Work out the finished part from the listing and answer in its coordinate system (mm). A direction names the side the tool comes from. Give positions to 0.01 mm unless a question says otherwise; leave off trailing zeros. Write each loop counter-clockwise with the first axis right and the second up, starting at its lowest first coordinate (ties: lowest second). Pieces come first, ordered by that corner, then holes.
1) A tool of negligible diameter and unlimited length cuts with its end or side. For faces 4 (the face through (-30.426, -17.744, 23.33)), 5 (the face through (-5.357, -7.513, 40.798)), 6 (the face through (0.553, -5.128, -34.887)), from which of +Z, -Z, +X, -X, +Y, -Y can it reach the whole face along a straight path? Write none if from no direction.
2) Given pin 1 Ø1 at (x, y) = (-2, -20.5) entering from -Z; pin 2 Ø3 at (x, y) = (-27, -12.5) entering from +Z; pin 3 Ø24.5 at (x, z) = (-3, -19.5) entering from -Y, each flat-ended and moving along its own axis, determine where each tip first touches the part or whether it passes through.
3) Determine the mould class of faces 1 (the face through (10.19, -16.51, 23.45)), 2 (the face through (-27.24, -20.32, 27.24)), 3 (the face through (-5.357, -22.824, 40.798)) for opening direction Y: pulls with the +Y half, pulls with the -Y half, needs draft (parallel to the pull), parting line crosses it, or undercut.
4) Find section A-A (x = 58). Determine the outline of the cut face in (y, z) (3 decimals), plus the area to 3 significant figures.
5) Straight lines are drawn through the part: probe 1 along Y at (x, z) = (0, -33.5) (3 decimals); probe 2 along Y at (x, z) = (-35.5, 48) (3 decimals); probe 3 along Y at (x, z) = (-23.5, -20.5) (3 decimals). For each, find the intervals that lie inside material, in ascending order.
6) Find section C-C (x = -57.15). Determine the outline of the cut face in (y, z) (3 decimals).
7) Find section B-B (z = 30). Determine the outline of the cut face in (x, y) (3 decimals).
```python
from build123d import *

# Parameters (mm, degrees)
SKETCH1_R                       = 66.675
SKETCH1_R_2                     = 20.32
BOSS_EXTRUDE1_DEPTH             = 4.445
F_1_4_0_25_DIAMETER_HOLE1_D     = 6.35
F_1_4_0_25_DIAMETER_HOLE1_DEPTH = 4.446
CIRPATTERN1_COUNT               = 6
SKETCH6_R                       = 41.148
SKETCH6_R_2                     = 20.32
BOSS_EXTRUDE2_DEPTH             = 25.4
SKETCH9_W                       = 2.9337
SKETCH9_H                       = 5.08
CIRPATTERN2_COUNT               = 6
F_3_32_0_09375_DIAMETER_HOLE1_D = 2.38125
SKETCH13_R                      = 34.925
CUT_EXTRUDE1_DEPTH              = 8.89
CHAMFER2_SIZE                   = 5.08


with BuildPart() as part:
    # Sketch1 → Boss-Extrude1 (new body)
    with BuildSketch(Plane(origin=(0, 0, 0), x_dir=(1, 0, 0), z_dir=(0, 1, 0))):
        Circle(SKETCH1_R)
        Circle(SKETCH1_R_2, mode=Mode.SUBTRACT)
    extrude(amount=BOSS_EXTRUDE1_DEPTH)

    # 1/4 (0.25) Diameter Hole1
    with Locations(Plane(origin=(0, 4.445, 0), x_dir=(1, 0, 0), z_dir=(0, 1, 0))):
        with Locations((57.15, 0)):
            f_1_4_0_25_diameter_hole1 = Hole(F_1_4_0_25_DIAMETER_HOLE1_D / 2, depth=F_1_4_0_25_DIAMETER_HOLE1_DEPTH)

    # CirPattern1: 1/4 (0.25) Diameter Hole1 ×6 about axis
    cirpattern1_axis = Axis((0, 0, 0), (0, 1, 0))
    for i in range(1, CIRPATTERN1_COUNT):
        add(f_1_4_0_25_diameter_hole1.rotate(cirpattern1_axis, i * 360 / CIRPATTERN1_COUNT), mode=Mode.SUBTRACT)

    # Sketch6 → Boss-Extrude2 (add)
    with BuildSketch(Plane.XZ):
        Circle(SKETCH6_R)
        Circle(SKETCH6_R_2, mode=Mode.SUBTRACT)
    extrude(amount=BOSS_EXTRUDE2_DEPTH)

    # Sketch9 → Cut-Revolve3 (revolve, cut)
    with BuildSketch(Plane.XY):
        with Locations((39.80815, -17.78)):
            Rectangle(SKETCH9_W, SKETCH9_H)
    revolve(axis=Axis((0, -0.47625, 0), (0, 1, 0)), mode=Mode.SUBTRACT)

    # Sketch10 → 1/4-20 Tapped Hole1 (revolve, cut)
    with BuildSketch(Plane(origin=(-35.635213315, -7.62, 20.574), x_dir=(0.5, 0, 0.866025404), z_dir=(0, 1, 0))):
        Polygon((0, 0), (0, 14.233816902), (2.5527, 12.7), (2.5527, 0), align=None)
    f_1_4_20_tapped_hole1 = revolve(axis=Axis((-41.134474629, -7.62, 23.749), (0.866025404, 0, -0.5)), mode=Mode.SUBTRACT)

    # CirPattern2: 1/4-20 Tapped Hole1 ×6 about axis
    cirpattern2_axis = Axis((0, -0.47625, 0), (0, 1, 0))
    for i in range(1, CIRPATTERN2_COUNT):
        add(f_1_4_20_tapped_hole1.rotate(cirpattern2_axis, i * 360 / CIRPATTERN2_COUNT), mode=Mode.SUBTRACT)

    # 3/32 (0.09375) Diameter Hole1 (through all)
    with Locations(Plane(origin=(0, 4.445, 0), x_dir=(1, 0, 0), z_dir=(0, 1, 0))):
        with Locations((31.75, 0)):
            Hole(F_3_32_0_09375_DIAMETER_HOLE1_D / 2)

    # Sketch13 → Cut-Extrude1 (cut)
    with BuildSketch(Plane.XZ.offset(25.4)):
        Circle(SKETCH13_R)
    extrude(amount=-CUT_EXTRUDE1_DEPTH, mode=Mode.SUBTRACT)

    # Chamfer2
    chamfer2_edges = [part.edges().sort_by_distance(p)[0] for p in [
        (-20.32, -16.51, 0),
    ]]
    chamfer(chamfer2_edges, length=CHAMFER2_SIZE)


solid = part.part
```
Results:
1. face 4: none
1. face 5: -Y
1. face 6: -Z
2. pin 1: stops at z = -41.12
2. pin 2: stops at z = 32.29
2. pin 3: stops at y = -16.51
3. face 1: pulls with the -Y half
3. face 2: undercut
3. face 3: needs draft
4. outline: (0, -32.887) - (4.445, -32.887) - (4.445, -3.059) - (0, -3.059) - close; (0, 3.059) - (4.445, 3.059) - (4.445, 32.887) - (0, 32.887) - close
4. area: 265 mm2
5. probe 1: y = -16.51 to -10.173, -5.067 to 4.445
5. probe 2: y = 0 to 4.445
5. probe 3: y = -16.51 to 4.445
6. outline: (0, -34.343) - (4.445, -34.343) - (4.445, -3.175) - (0, -3.175) - close; (0, 3.175) - (4.445, 3.175) - (4.445, 34.343) - (0, 34.343) - close
7. outline: (-59.545, 0) - (-28.163, 0) - (-28.163, -15.24) - (-23.876, -15.24) - (-23.876, -20.32) - (-28.163, -20.32) - (-28.163, -25.4) - (-17.882, -25.4) - (-17.882, -16.51) - (17.882, -16.51) - (17.882, -25.4) - (28.163, -25.4) - (28.163, -20.32) - (23.876, -20.32) - (23.876, -15.24) - (28.163, -15.24) - (28.163, 0) - (59.545, 0) - (59.545, 4.445) - (-59.545, 4.445) - close; hole circle Ø5.105 at (0, -7.62)
